The listing builds one solid part. Answer for the finished solid, in the listing's coordinates (mm). A direction names the side the tool comes from. Give positions to 0.01 mm unless a question says otherwise; leave off trailing zeros. Loops run counter-clockwise (first coordinate to the right, second up) from the corner with the lowest first, then second, coordinate; pieces in that order, holes last.
Item 1: A tool of negligible diameter and unlimited length cuts with its end or side. For faces 4 (the face through (-13.887, -10.648, 27.185)), 5 (the face through (-70, 0, 2)), from which of +Z, -Z, +X, -X, +Y, -Y can it reach the whole face along a straight path? Write none if from no direction.
Item 2: Section C-C, the plane y = 0 is taken. Give the vertices of the cut face in (x, z).
Item 3: Section D-D, the plane z = 104 is taken. Give the vertices of the cut face in (x, y), and give its area (3 significant figures).
Item 4: Consider line 1 along Y through (x, z) = (-45, 2.8); line 2 along Z through (x, y) = (58.5, 10.5); line 3 along Z through (x, y) = (-16.5, -2.5). Determine where each line is inside the solid, lowest interval first.
Item 5: Section A-A, the plane x = 45 is taken. Give the vertices of the cut face in (y, z), and give its area (3 significant figures).
Item 6: Section B-B, the plane x = 0 is taken. Give the vertices of the cut face in (y, z).
Item 7: Each of these flat-tipped pins is pushed along its axis until it touches: pin 1 Ø11 at (x, y) = (45, 16) entering from -Z; pin 2 Ø18 at (x, y) = (33, -11.5) entering from +Z; pin 3 Ø4 at (x, z) = (4.5, 107) entering from +Y; pin 4 Ø3 at (x, z) = (-7.5, 18) entering from +Y. Where does it stop, or does it pass through?
Item 8: The mould has two halves that part along X. Classify faces 1 (the face through (-7.493, 0.33, 91.905)), 2 (the face through (-51, 16, 2)), 3 (the face through (0, -8, 50)): pulls with the +X half, pulls with the -X half, needs draft (parallel to the pull), parting line crosses it, or undercut.
from build123d import *

# Parameters (mm, degrees)
SKETCH1_W           = 140
SKETCH1_H           = 60
SKETCH1_R           = 6
BOSS_EXTRUDE1_DEPTH = 5
SKETCH2_R           = 17.5
BOSS_EXTRUDE2_DEPTH = 45
SKETCH3_R           = 7.5
BOSS_EXTRUDE3_DEPTH = 85


with BuildPart() as part:
    # Sketch1 → Boss-Extrude1 (new body)
    with BuildSketch(Plane.XY):
        Rectangle(SKETCH1_W, SKETCH1_H)
        with Locations((-45, 16)):
            Circle(SKETCH1_R, mode=Mode.SUBTRACT)
        with Locations((-45, -16)):
            Circle(SKETCH1_R, mode=Mode.SUBTRACT)
        with Locations((45, -16)):
            Circle(SKETCH1_R, mode=Mode.SUBTRACT)
        with Locations((45, 16)):
            Circle(SKETCH1_R, mode=Mode.SUBTRACT)
    extrude(amount=BOSS_EXTRUDE1_DEPTH)

    # Sketch2 → Boss-Extrude2 (add)
    with BuildSketch(Plane.XY.offset(5)):
        Circle(SKETCH2_R)
    extrude(amount=BOSS_EXTRUDE2_DEPTH)

    # Sketch3 → Boss-Extrude3 (add)
    with BuildSketch(Plane.XY.offset(50)):
        Circle(SKETCH3_R)
    extrude(amount=BOSS_EXTRUDE3_DEPTH)


solid = part.part
Worked answers:
1. face 4: +Z
1. face 5: +Z, -Z, -X, +Y, -Y
2. outline: (-70, 0) - (70, 0) - (70, 5) - (17.5, 5) - (17.5, 50) - (7.5, 50) - (7.5, 135) - (-7.5, 135) - (-7.5, 50) - (-17.5, 50) - (-17.5, 5) - (-70, 5) - close
3. outline: circle Ø15 at (0, 0)
3. area: 177 mm2
4. line 1: y = -30 to -22, -10 to 10, 22 to 30
4. line 2: z = 0 to 5
4. line 3: z = 0 to 50
5. outline: (-30, 0) - (-22, 0) - (-22, 5) - (-30, 5) - close; (-10, 0) - (10, 0) - (10, 5) - (-10, 5) - close; (22, 0) - (30, 0) - (30, 5) - (22, 5) - close
5. area: 180 mm2
6. outline: (-30, 0) - (30, 0) - (30, 5) - (17.5, 5) - (17.5, 50) - (7.5, 50) - (7.5, 135) - (-7.5, 135) - (-7.5, 50) - (-17.5, 50) - (-17.5, 5) - (-30, 5) - close
7. pin 1: passes through
7. pin 2: stops at z = 5
7. pin 3: stops at y = 7.07
7. pin 4: stops at y = 16.44
8. face 1: parting line crosses it
8. face 2: undercut
8. face 3: needs draft
